Geometry check sheet. Reference: the model listing, model coordinates, mm. Round coordinates to 2 decimals unless told otherwise and drop trailing zeros. Order: outer loops, then holes, each group sorted by start corner. A loop starts at its lowest first (then second) coordinate and runs counter-clockwise, first axis right, second up. Notation, with made-up numbers: (53.5, 33) -> (96.5, 33) arc R26 cw to (96.5, 51) -> close; hole circle Ø1 at (14.5, 5). An arc over 180 degrees is marked (long way). Use a Markdown table: item, result. Add a question column.
Item 1: Sectioned sample at B-B, the plane y = 69.85. Record the cut outline in (x, z), and give its area (3 significant figures).
Item 2: Sectioned sample at A-A, the plane x = -97.79. Record the cut outline in (y, z), and give its area (3 significant figures).
Item 3: Material ranges on probe 1 along X at (y, z) = (34.5, 3.5); probe 2 along Y at (x, z) = (-97.79, 2.5); probe 3 along X at (y, z) = (111, 4.5), recorded low to high. Write a range as [from, to].
Item 4: Sectioned sample at C-C, the plane z = 1. Record the cut outline in (x, y).
Item 5: Gauge pin test, flat end, axial feed: pin 1 Ø14 at (x, y) = (97.79, 112.58) entering from +Z. Record the tip position at first contact, or that the pin passes through.
Item 6: Mould release check, pull along X, two halves, no side actions. Record for faces 1 (the flat face through (151.892, 79, 3)), 2 (the flat face through (127, 30.033, 3)), 3 (the cylindrical face through (-97.908, 39.647, 3.131)): pulls with the +X half, pulls with the -X half, needs draft (parallel to the pull), parting line crosses it, or undercut.
from build123d import *

# Parameters (mm, degrees)
BOSS_EXTRUDE1_DEPTH              = 6.35
CUT_EXTRUDE3_DEPTH               = 221.472033966
F_27_64_0_42188_DIAMETER_HOLE1_D = 10.715752
FILLET1_R                        = 2.54
F_1_2_CLEARANCE_HOLE1_D          = 13.49248
SKETCH7_W                        = 303.784
SKETCH7_H                        = 55.43328257
CUT_EXTRUDE1_DEPTH               = 200.030230178
CUT_EXTRUDE2_DEPTH               = 200.030230178
FILLET2_R                        = 2.54


with BuildPart() as part:
    # Sketch1 → Boss-Extrude1 (new body)
    with BuildSketch(Plane.XY):
        with BuildLine():
            Line((-179.07, -25.4), (-179.07, 128.45828257))
            Line((-179.07, 128.45828257), (179.07, 128.45828257))
            Line((179.07, 128.45828257), (179.07, -25.4))
            Line((179.07, -25.4), (153.67, -25.4))
            Line((153.67, -25.4), (153.67, -1.27))
            ThreePointArc((153.67, -1.27), (127, 25.4), (100.33, -1.27))
            Line((100.33, -1.27), (100.33, -25.4))
            Line((100.33, -25.4), (-100.33, -25.4))
            Line((-100.33, -25.4), (-100.33, -1.27))
            ThreePointArc((-100.33, -1.27), (-127, 25.4), (-153.67, -1.27))
            Line((-153.67, -1.27), (-153.67, -25.4))
            Line((-153.67, -25.4), (-179.07, -25.4))
        make_face()
    extrude(amount=BOSS_EXTRUDE1_DEPTH)

    # Sketch9 → Cut-Extrude3 (cut, through all)
    with BuildSketch(Plane.XY.offset(6.35)):
        with BuildLine():
            Line((-151.892, 128.45828257), (-151.892, 8.304823027))
            ThreePointArc((-151.892, 8.304823027), (-153.22173278, 3.599253536), (-153.67, -1.27))
            Line((-153.67, -1.27), (-153.67, -25.4))
            Line((-153.67, -25.4), (-179.07, -25.4))
            Line((-179.07, -25.4), (-179.07, 128.45828257))
            Line((-179.07, 128.45828257), (-151.892, 128.45828257))
        make_face()
        with BuildLine():
            Line((153.67, -25.4), (153.67, -1.27))
            ThreePointArc((153.67, -1.27), (153.22173278, 3.599253536), (151.892, 8.304823027))
            Line((151.892, 8.304823027), (151.892, 128.45828257))
            Line((151.892, 128.45828257), (179.07, 128.45828257))
            Line((179.07, 128.45828257), (179.07, -25.4))
            Line((179.07, -25.4), (153.67, -25.4))
        make_face()
    extrude(amount=-CUT_EXTRUDE3_DEPTH, mode=Mode.SUBTRACT)

    # 27/64 (0.42188) Diameter Hole1 (through all)
    with Locations(Plane.XY.offset(6.35)):
        with Locations((-97.79, 34.29), (-97.79, 112.58328257), (97.79, 34.29), (97.79, 112.58328257)):
            Hole(F_27_64_0_42188_DIAMETER_HOLE1_D / 2)

    # Fillet1
    fillet1_edges = [part.edges().sort_by_distance(p)[0] for p in [
        (100.33, -25.4, 3.175),
        (-100.33, -25.4, 3.175),
        (-151.892, 128.45828257, 3.175),
        (-151.892, 8.304823027, 3.175),
        (151.892, 8.304823027, 3.175),
        (151.892, 128.45828257, 3.175),
    ]]
    fillet(fillet1_edges, radius=FILLET1_R)

    # 1/2 Clearance Hole1 (through all)
    with Locations(Plane.XY.offset(6.35)):
        with Locations((57.15, 69.85), (-57.15, 69.85)):
            Hole(F_1_2_CLEARANCE_HOLE1_D / 2)

    # Sketch7 → Cut-Extrude1 (cut, through all)
    with BuildSketch(Plane.XY.offset(6.35)):
        with Locations((0, 2.316641285)):
            Rectangle(SKETCH7_W, SKETCH7_H)
    extrude(amount=-CUT_EXTRUDE1_DEPTH, mode=Mode.SUBTRACT)

    # Sketch8 → Cut-Extrude2 (cut, through all)
    with BuildSketch(Plane.XY.offset(6.35)):
        Polygon((-94.536203455, 30.03328257), (-92.432124, 30.03328257), (-92.432124, 34.29), align=None)
        Polygon((-103.147876, 34.29), (-103.147876, 30.03328257), (-101.043796545, 30.03328257), align=None)
        Polygon((101.043796545, 30.03328257), (103.147876, 30.03328257), (103.147876, 34.29), align=None)
        Polygon((92.432124, 34.29), (92.432124, 30.03328257), (94.536203455, 30.03328257), align=None)
    extrude(amount=-CUT_EXTRUDE2_DEPTH, mode=Mode.SUBTRACT)

    # Fillet2
    fillet2_edges = [part.edges().sort_by_distance(p)[0] for p in [
        (-151.892, 30.03328257, 3.175),
        (151.892, 30.03328257, 3.175),
        (-103.147876, 30.03328257, 3.175),
        (103.147876, 30.03328257, 3.175),
        (92.432124, 30.03328257, 3.175),
        (-92.432124, 30.03328257, 3.175),
    ]]
    fillet(fillet2_edges, radius=FILLET2_R)


solid = part.part
Found:
| question | item | result |
|---|---|---|
| 1 | outline | (-151.89, 0) -> (-63.9, 0) -> (-63.9, 6.35) -> (-151.89, 6.35) -> close; (-50.4, 0) -> (50.4, 0) -> (50.4, 6.35) -> (-50.4, 6.35) -> close; (63.9, 0) -> (151.89, 0) -> (151.89, 6.35) -> (63.9, 6.35) -> close |
| 1 | area | 1,760 mm2 |
| 2 | outline | (39.65, 0) -> (107.23, 0) -> (107.23, 6.35) -> (39.65, 6.35) -> close; (117.94, 0) -> (128.46, 0) -> (128.46, 6.35) -> (117.94, 6.35) -> close |
| 2 | area | 496 mm2 |
| 3 | probe 1 | x = [-151.89, -103.14], [-92.44, 92.44], [103.14, 151.89] |
| 3 | probe 2 | y = [39.65, 107.23], [117.94, 128.46] |
| 3 | probe 3 | x = [-151.89, -102.91], [-92.67, 92.67], [102.91, 151.89] |
| 4 | outline | (-151.89, 32.57) arc R2.54 ccw to (-149.35, 30.03) -> (-105.69, 30.03) arc R2.54 ccw to (-103.15, 32.57) -> (-103.15, 34.29) arc R5.36 cw to (-92.43, 34.29) -> (-92.43, 32.57) arc R2.54 ccw to (-89.89, 30.03) -> (89.89, 30.03) arc R2.54 ccw to (92.43, 32.57) -> (92.43, 34.29) arc R5.36 cw to (103.15, 34.29) -> (103.15, 32.57) arc R2.54 ccw to (105.69, 30.03) -> (149.35, 30.03) arc R2.54 ccw to (151.89, 32.57) -> (151.89, 125.92) arc R2.54 ccw to (149.35, 128.46) -> (-149.35, 128.46) arc R2.54 ccw to (-151.89, 125.92) -> close; hole circle Ø10.72 at (-97.79, 112.58); hole circle Ø13.49 at (-57.15, 69.85); hole circle Ø13.49 at (57.15, 69.85); hole circle Ø10.72 at (97.79, 112.58) |
| 5 | pin 1 | stops at z = 6.35 |
| 6 | face 1 | pulls with the +X half |
| 6 | face 2 | needs draft |
| 6 | face 3 | undercut |
